Autodesk Inventor part; units mm, degrees
ref_plane "YZ Plane" through (0, 0, 0) normal (1, 0, 0) x (0, 1, 0)
ref_plane "XZ Plane" through (0, 0, 0) normal (0, 1, 0) x (-1, 0, 0)
ref_plane "XY Plane" through (0, 0, 0) normal (0, 0, 1) x (1, 0, 0)
sketch "Sketch1" plane through (0, 0, 0) normal (1, 0, 0) x (0, 1, 0)
  circle A0 centre (0, 0) radius 2.5
  dimension "d0" = 5
extrude "Extrusion1" add sketch "Sketch1" along normal blind 100
sketch "Sketch2" plane through (0, 0, 0) normal (-1, 0, 0) x (0, 0, 1)
  point P0 (0, 0)
sketch "Sketch3" plane through (0, 0, 0) normal (-1, 0, 0) x (0, 0, 1)
  point P0 (0, 0)
sketch "Sketch4" plane through (0, 0, 0) normal (0, 0, 1) x (1, 0, 0)
  circle A0 centre (44.8186, 0) radius 1.5
  point P0 (0, 0)
  dimension "d3" = 3
extrude "Extrusion2" add sketch "Sketch4" along normal blind 8
sketch "Sketch5" plane through (44.8186, 0, 8) normal (0, 0, 1) x (1, 0, 0)
  circle A0 centre (0, 0) radius 2.5
  point P0 (-44.8186, 0)
  dimension "d6" = 5
extrude "Extrusion3" add sketch "Sketch5" against normal blind 2
properties part number "stylo part1"
Model file for the job. Use its own axes, mm. A direction names the side the tool comes from. Coordinates: 2 decimals unless noted, no trailing zeros. Loops run counter-clockwise (first coordinate to the right, second up) from the corner with the lowest first, then second, coordinate; pieces in that order, holes last. Notation, with made-up numbers: (-27.75, 52.25) -> (15.25, 52.25) arc R12 ccw to (15.25, 71.25) -> close; hole circle Ø9 at (86.5, 21). An arc over 180 degrees is marked (long way). Answer as a JSON object with one key per item and string values.
Q1. Flat gauge pins, fed straight in: P1, Ø2, axis at x = 79, y = 1, coming from the +Z side; P2, Ø1, axis at x = 36, y = -1, coming from the +Z side; P3, Ø1, axis at x = 59.5, z = 2, coming from the -Y side; P4, Ø6, axis at x = 47.5, z = 6.5, coming from the +Y side. Where does each tip first touch, or does it go through?
Report:
{"P1": "stops at z = 2.5", "P2": "stops at z = 2.45", "P3": "stops at y = -2", "P4": "stops at y = 2.5"}
Q2. Probe probe 1 along Z at (x, y) = (25, -0.05); probe 2 along Z at (x, y) = (78, -1.55); probe 3 along Y at (x, z) = (88, -2). List the from-to ranges inside material, lowest first.
Report:
{"probe 1": "z = -2.5 to 2.5", "probe 2": "z = -1.96 to 1.96", "probe 3": "y = -1.5 to 1.5"}
Q3. Cut at B-B (z = 7). List the corners of the cut face in (x, y).
Report:
{"outline": "circle Ø5 at (44.82, 0)"}
Q4. Cut at D-D (z = 1). List the corners of the cut face in (x, y), and give its area (3 significant figures).
Report:
{"outline": "(0, -2.29) -> (100, -2.29) -> (100, 2.29) -> (0, 2.29) -> close", "area": "458 mm2"}
Q5. Cut at A-A (y = 0). List the corners of the cut face in (x, z).
Report:
{"outline": "(0, -2.5) -> (100, -2.5) -> (100, 2.5) -> (46.32, 2.5) -> (46.32, 6) -> (47.32, 6) -> (47.32, 8) -> (42.32, 8) -> (42.32, 6) -> (43.32, 6) -> (43.32, 2.5) -> (0, 2.5) -> close"}
Q6. 3-axis set-ups, long thin cutter, end or side, ignore diameter. For faces 4 (the flat face through (100, 0, 0)), 5 (the cylindrical face through (47.128, -0.958, 7.014)), 6 (the flat face through (45, -2, 6)): which of +Z, -Z, +X, -X, +Y, -Y reach the whole face in a straight line?
Report:
{"face 4": "+Z, -Z, +X, +Y, -Y", "face 5": "+Z", "face 6": "none"}
Q7. Cut at C-C (x = 50). List the corners of the cut face in (y, z), and give its area (3 significant figures).
Report:
{"outline": "circle Ø5 at (0, 0)", "area": "19.6 mm2"}
Q8. Pull direction Z, two halves, no side cores. Call faces 1 (the flat face through (45, 0, 8)), 2 (the cylindrical face through (46.25, -0.45, 3.97)), 3 (the flat face through (0, 0, 0)): released by +Z, released by -Z, zero draft, split by the parting line, or undercut.
Report:
{"face 1": "released by +Z", "face 2": "undercut", "face 3": "zero draft"}
